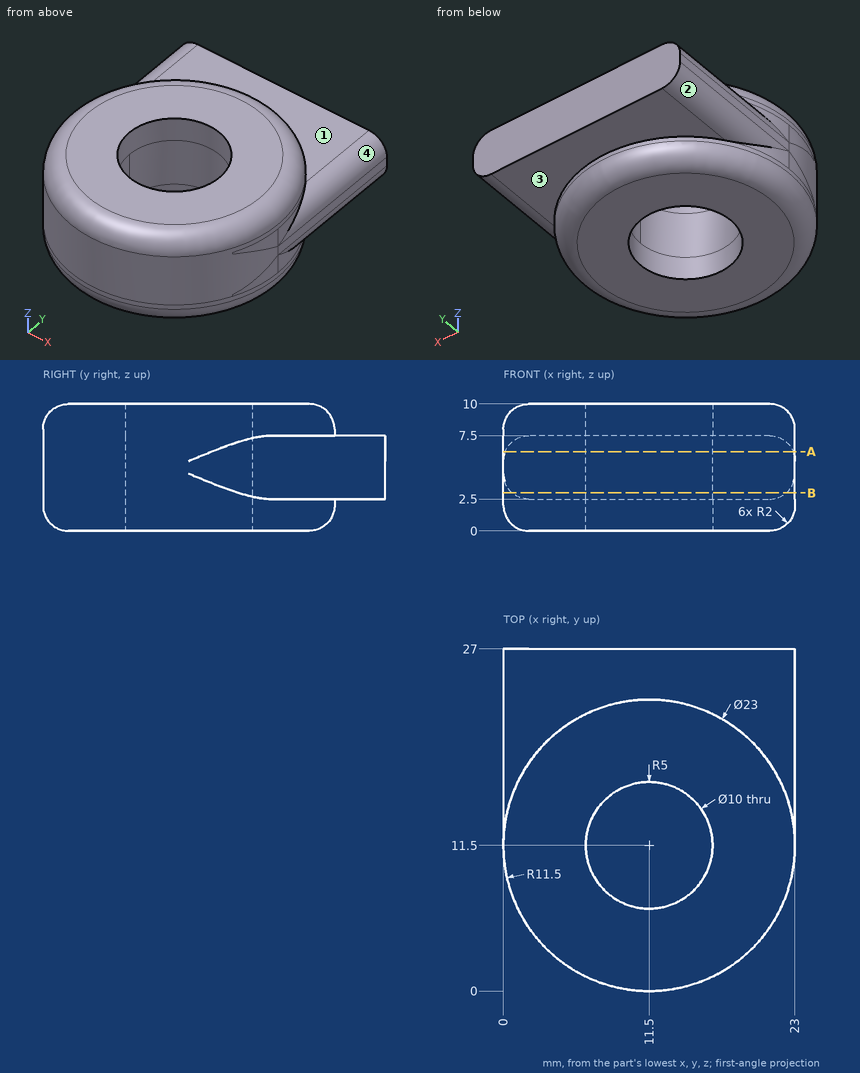
The figure shows three views and two pictorial views of one solid part (mm, origin at its lowest corner). Answer the questions. A direction names the side the tool comes from. Round coordinates to 2 decimals unless told otherwise and drop trailing zeros. Order: outer loops, then holes, each group sorted by start corner. A loop starts at its lowest first (then second) coordinate and runs counter-clockwise, first axis right, second up.
Q1. Given pin 1 Ø1 at (x, z) = (5, 3.5) entering from -Y; pin 2 Ø1 at (y, z) = (5.5, 5.5) entering from -X; pin 3 Ø1.5 at (x, z) = (3.5, 6) entering from -Y, each flat-ended and moving along its own axis, determine where each tip first touches the part or whether it passes through.
Solution:
pin 1: stops at y = 1.69
pin 2: stops at x = 1.4
pin 3: stops at y = 2.57
Q2. A tool of negligible diameter and unlimited length cuts with its end or side. For the marked faces 1, 2, 3 and 4, from which of +Z, -Z, +X, -X, +Y, -Y can it reach the whole face along a straight path? Write none if from no direction.
Solution:
face 1: +Z, +Y
face 2: -Z, -X, +Y
face 3: -Z, +Y
face 4: +Z, +X, +Y
Q3. Find the intervals of material crossed by line 1 along X through (y, z) = (11.75, 4.75); line 2 along Y through (x, z) = (15.25, 9.25); line 3 along Y through (x, z) = (16, 2.25), in increasing order.
Solution:
line 1: x = 0 to 6.51, 16.49 to 23
line 2: y = 1.09 to 8.19, 14.81 to 21.91
line 3: y = 0.92 to 9.32, 13.68 to 22.08
Q4. A cutting plane is placed at B-B, the plane z = 3. Determine the outline of the cut face in (x, y).
Solution:
outline: (0.68, 15.39) arc R11.5 ccw (long way) to (22.32, 15.39) - (22.32, 27) - (0.68, 27) - close; hole circle Ø10 at (11.5, 11.5)
Q5. A cutting plane is placed at A-A, the plane z = 6.25. Determine the outline of the cut face in (x, y).
Solution:
outline: (0.15, 13.33) arc R11.5 ccw (long way) to (22.85, 13.33) - (22.85, 27) - (0.15, 27) - close; hole circle Ø10 at (11.5, 11.5)
